Read the model definition and answer for the solid it produces. Units are mm, in the model's axes. Give positions to 0.01 mm unless a question says otherwise; leave off trailing zeros. Write each loop counter-clockwise with the first axis right and the second up, starting at its lowest first coordinate (ties: lowest second). Pieces come first, ordered by that corner, then holes. Notation, with made-up numbers: (-25.5, 69.25) -> (31.5, 69.25) arc R10 cw to (31.5, 87.25) -> close; hole circle Ø3 at (80.25, -7.75). An arc over 180 degrees is marked (long way). Write item = value, one per line.
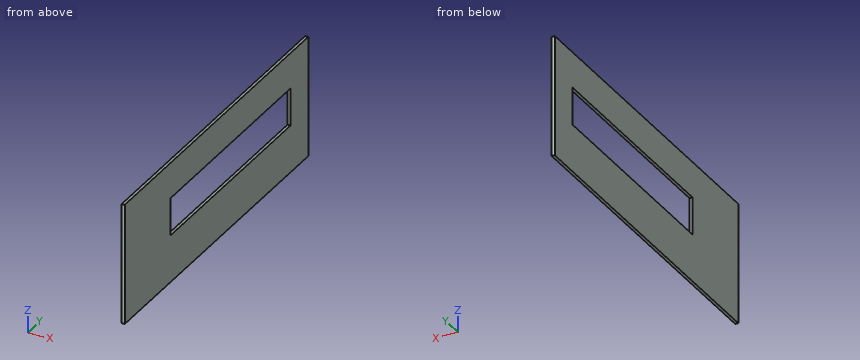
from build123d import *

# Parameters (mm, degrees)
SKETCH_1_W          = 110.7
SKETCH_1_H          = 38.85
EXTRUDE_1_DEPTH     = 1
SKETCH_2_W          = 12.12
SKETCH_2_H          = 72.46
CUT_EXTRUDE_1_DEPTH = 10


with BuildPart() as part:
    # Эскиз1 → Бобышка-Вытянуть1 (new body)
    with BuildSketch(Plane(origin=(0.5, 0, 0), x_dir=(0, -1, 0), z_dir=(-1, 0, 0))):
        with Locations((-45.5, 22.825)):
            Rectangle(SKETCH_1_W, SKETCH_1_H)
    extrude(amount=-EXTRUDE_1_DEPTH)

    # Эскиз2 → Вырез-Вытянуть1 (cut)
    with BuildSketch(Plane.ZY.offset(-0.5)):
        with Locations((24.69, 53.98)):
            Rectangle(SKETCH_2_W, SKETCH_2_H)
    extrude(amount=-CUT_EXTRUDE_1_DEPTH, mode=Mode.SUBTRACT)


solid = part.part
(1) Consider L1, parallel to Y at x = 0.8, z = 20; L2, parallel to Z at x = 0.9, y = 39.5. Determine where each line is inside the solid, lowest interval first.
Checks:
L1 = -9.85 to 17.75, 90.21 to 100.85
L2 = 3.4 to 18.63, 30.75 to 42.25
(2) The part is cut by section C-C on x = 1. Determine the outline of the cut face in (y, z), plus the area to 3 significant figures.
Checks:
outline = (-9.85, 3.4) -> (100.85, 3.4) -> (100.85, 42.25) -> (-9.85, 42.25) -> close; hole (17.75, 18.63) -> (90.21, 18.63) -> (90.21, 30.75) -> (17.75, 30.75) -> close
area = 3,420 mm²
(3) The part is cut by section B-B on y = 70. Determine the outline of the cut face in (x, z), plus the area to 3 significant figures.
Checks:
outline = (0.5, 3.4) -> (1.5, 3.4) -> (1.5, 18.63) -> (0.5, 18.63) -> close; (0.5, 30.75) -> (1.5, 30.75) -> (1.5, 42.25) -> (0.5, 42.25) -> close
area = 26.7 mm²
(4) Given P1, Ø1.5, axis at y = 20.5, z = 20.5, coming from the -X side, flat-ended and moving along its own axis, determine where the tip first touches the part or whether it passes through.
Checks:
P1 = through
(5) The part is cut by section A-A on z = 21.5. Determine the outline of the cut face in (x, y), plus the area to 3 significant figures.
Checks:
outline = (0.5, -9.85) -> (1.5, -9.85) -> (1.5, 17.75) -> (0.5, 17.75) -> close; (0.5, 90.21) -> (1.5, 90.21) -> (1.5, 100.85) -> (0.5, 100.85) -> close
area = 38.2 mm²
